The listing builds one solid part. Answer for the finished solid, in the listing's coordinates (mm). Give positions to 0.01 mm unless a question says otherwise; leave off trailing zeros. Write each loop counter-clockwise with the first axis right and the second up, starting at its lowest first coordinate (ties: lowest second). Pieces come first, ordered by that corner, then holes.
Solid Edge part; units mm, degrees
sketch "Sketch1" plane through (0, 0, 8) normal (0, 0, 1) x (1, 0, 0)
  line L0 (-28, -49) -> (28, -49)
  line L1 (28, -49) -> (28, 24)
  line L2 (28, 24) -> (-28, 24)
  line L3 (-28, 24) -> (-28, -49)
  circle A0 centre (0, 0) radius 12
  circle A1 centre (11.3137, 11.3137) radius 1.7
  circle A2 centre (-11.3137, 11.3137) radius 1.7
  circle A3 centre (-11.3137, -11.3137) radius 1.7
  circle A4 centre (11.3137, -11.3137) radius 1.7
  circle A5 centre (-23, -43) radius 1.7
  circle A6 centre (23, -43) radius 1.7
  circle A7 centre (-23, 18) radius 1.7
  circle A8 centre (23, 18) radius 1.7
extrude "ExtrudedProtrusion_1" add sketch "Sketch1" along normal blind 4
Item 1: Determine the mould class of faces 1 (the face through (23.8, -41.5, 10)), 2 (the face through (28, -13, 10)), 3 (the face through (-7, -12, 8)) for opening direction X: pulls with the +X half, pulls with the -X half, needs draft (parallel to the pull), parting line crosses it, or undercut.
Conclusion:
face 1: undercut
face 2: pulls with the +X half
face 3: needs draft
Item 2: Consider probe 1 along Y at (x, z) = (23, 8.9); probe 2 along Y at (x, z) = (0, 10.5); probe 3 along X at (y, z) = (6.5, 11.15). Determine where each line is inside the solid, lowest interval first.
Conclusion:
probe 1: y = -49 to -44.7, -41.3 to 16.3, 19.7 to 24
probe 2: y = -49 to -12, 12 to 24
probe 3: x = -28 to -10.09, 10.09 to 28
Item 3: A cutting plane is placed at B-B, the plane x = -23. Give the vertices of the cut face in (y, z).
Conclusion:
outline: (-49, 8) - (-44.7, 8) - (-44.7, 12) - (-49, 12) - close; (-41.3, 8) - (16.3, 8) - (16.3, 12) - (-41.3, 12) - close; (19.7, 8) - (24, 8) - (24, 12) - (19.7, 12) - close
Item 4: A cutting plane is placed at C-C, the plane y = -3. Give the vertices of the cut face in (x, z), plus the area to 3 significant figures.
Conclusion:
outline: (-28, 8) - (-11.62, 8) - (-11.62, 12) - (-28, 12) - close; (11.62, 8) - (28, 8) - (28, 12) - (11.62, 12) - close
area: 131 mm2
Item 5: Each of these flat-tipped pins is pushed along its axis until it touches: P1, Ø5.5, axis at x = 23, y = 18, coming from the -Z side; P2, Ø21.5, axis at x = 0, y = 0, coming from the +Z side. Where does it stop, or does it pass through?
Conclusion:
P1: stops at z = 8
P2: passes through
Item 6: A cutting plane is placed at A-A, the plane y = -43. Give the vertices of the cut face in (x, z), plus the area to 3 significant figures.
Conclusion:
outline: (-28, 8) - (-24.7, 8) - (-24.7, 12) - (-28, 12) - close; (-21.3, 8) - (21.3, 8) - (21.3, 12) - (-21.3, 12) - close; (24.7, 8) - (28, 8) - (28, 12) - (24.7, 12) - close
area: 197 mm2
Item 7: A cutting plane is placed at D-D, the plane z = 11.2. Count the separate pieces of the cut face and the enclosed holes in it, plus the area to 3 significant figures.
Conclusion:
separate pieces: 1
enclosed holes: 9
area: 3,560 mm2
